Part print with two shaded views. Sizes in mm from the minimum x, y, z corner. Round coordinates to 2 decimals unless told otherwise and drop trailing zeros. Loops run counter-clockwise (first coordinate to the right, second up) from the corner with the lowest first, then second, coordinate; pieces in that order, holes last.
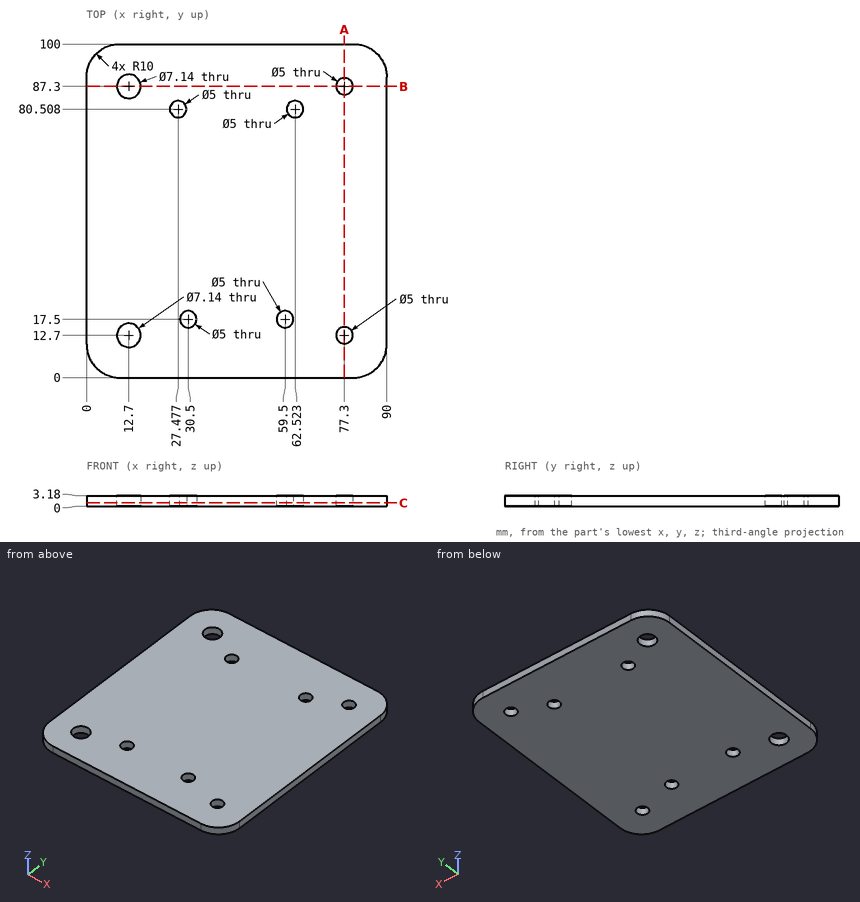
Item 1: Cut at A-A (x = 77.3). List the corners of the cut face in (y, z), plus the area to 3 significant figures.
Verdict:
outline: (0, 0) - (10.2, 0) - (10.2, 3.18) - (0, 3.18) - close; (15.2, 0) - (84.8, 0) - (84.8, 3.18) - (15.2, 3.18) - close; (89.8, 0) - (100, 0) - (100, 3.18) - (89.8, 3.18) - close
area: 286 mm2
Item 2: Wall check: L1, parallel to Y at x = 77.3, z = 0.8; L2, parallel to Y at x = 30.5, z = 0.95; L3, parallel to Y at x = 10, z = 0.9 (1 decimal). Give the ranges that are in metal, low to high.
Verdict:
L1: y = 0 to 10.2, 15.2 to 84.8, 89.8 to 100
L2: y = 0 to 15, 20 to 100
L3: y = 0 to 10.4, 15 to 85, 89.6 to 100
Item 3: Cut at B-B (y = 87.3). List the corners of the cut face in (x, z).
Verdict:
outline: (0, 0) - (9.13, 0) - (9.13, 3.18) - (0, 3.18) - close; (16.27, 0) - (74.8, 0) - (74.8, 3.18) - (16.27, 3.18) - close; (79.8, 0) - (90, 0) - (90, 3.18) - (79.8, 3.18) - close
Item 4: Cut at C-C (z = 1). State how many separate pieces and enclosed holes the cut face has, plus the area to 3 significant figures.
Verdict:
separate pieces: 1
enclosed holes: 8
area: 8,720 mm2
